from build123d import *

# Parameters (mm, degrees)
F0_R          = 6.35
F1_DEPTH      = 25.4
F2_W          = 19.05
F2_H          = 9.525
F3_DEPTH      = 25.401
F3_DEPTH_BACK = 25.401


with BuildPart() as f1:
    # F0 (on Top) → F1 (new body)
    with BuildSketch(Plane.XY):
        with BuildLine():
            Line((-34.925, -25.4), (34.925, -25.4))
            ThreePointArc((34.925, -25.4), (37.170064, -24.470064), (38.1, -22.225))
            Line((38.1, -22.225), (38.1, 22.225))
            ThreePointArc((38.1, 22.225), (37.170064, 24.470064), (34.925, 25.4))
            Line((34.925, 25.4), (-34.925, 25.4))
            ThreePointArc((-34.925, 25.4), (-37.170064, 24.470064), (-38.1, 22.225))
            Line((-38.1, 22.225), (-38.1, -22.225))
            ThreePointArc((-38.1, -22.225), (-37.170064, -24.470064), (-34.925, -25.4))
        make_face()
        Circle(F0_R, mode=Mode.SUBTRACT)
    extrude(amount=F1_DEPTH)

    # F2 (on Front) → F3 (cut, two sides)
    with BuildSketch(Plane.XZ) as f3_sk:
        with Locations((28.575, 20.6375)):
            Rectangle(F2_W, F2_H)
    extrude(amount=F3_DEPTH, mode=Mode.SUBTRACT)
    extrude(f3_sk.sketch, amount=-F3_DEPTH_BACK, mode=Mode.SUBTRACT)


solid = f1.part
Here's how the part is built. I have some questions about the finished solid (model axes, mm). A direction names the side the tool comes from. Give positions to 0.01 mm unless a question says otherwise; leave off trailing zeros. Order: outer loops, then holes, each group sorted by start corner. A loop starts at its lowest first (then second) coordinate and runs counter-clockwise, first axis right, second up. Notation, with made-up numbers: (71, 35) -> (85, 35) arc R19 cw to (85, 58) -> close; hole circle Ø4 at (-9, 80.5). An arc over 180 degrees is marked (long way). One line per item, written item: value. Start each with the question number.
1. Imagine slicing it at D-D, the plane y = -11. List the corners of the cut face in (x, z) for me (3 decimals).
2. Imagine slicing it at B-B, the plane y = 0. List the corners of the cut face in (x, z) for me (3 decimals).
3. For faces 5 (the face through (37.15, -24.49, 7.83)), 6 (the face through (19.05, 0, 21)), which set-ups out of +Z, -Z, +X, -X, +Y, -Y let a thin tool reach every point of the face, with its end or its side?
4. Will these pins go through, and if not, where does the flat tip stop? pin 1 Ø3 at (y, z) = (2.5, 20.5) entering from +X; pin 2 Ø9.5 at (x, y) = (25.5, -1.5) entering from +Z (3 decimals); pin 3 Ø4 at (x, z) = (21.5, 18.5) entering from -Y.
5. Imagine slicing it at C-C, the plane x = 5. List the corners of the cut face in (y, z) for me, plus the area to 3 significant figures.
6. We'd pull the mould along X, two halves only. Please class faces 1 (the face through (38.1, 0, 8)), 2 (the face through (-1.38, -6.2, 12.52)), 3 (the face through (-37.15, 24.49, 12.52)), 4 (the face through (-10, 0, 25.4)): released by +X, released by -X, zero draft, split by the parting line, or undercut.
7. I need wall thicknesses on probe 1 along Y at (x, z) = (0, 19.75); probe 2 along X at (y, z) = (22.5, 7.5); probe 3 along Z at (x, y) = (24.5, -3) (3 decimals). Which ranges of each line are inside material? Lowest first, please. Write a range as from..to.
8. Imagine slicing it at A-A, the plane z = 13. List the corners of the cut face in (x, y) for me (3 decimals).
Values follow:
1. outline: (-38.1, 0) -> (38.1, 0) -> (38.1, 15.875) -> (19.05, 15.875) -> (19.05, 25.4) -> (-38.1, 25.4) -> close
2. outline: (-38.1, 0) -> (-6.35, 0) -> (-6.35, 25.4) -> (-38.1, 25.4) -> close; (6.35, 0) -> (38.1, 0) -> (38.1, 15.875) -> (19.05, 15.875) -> (19.05, 25.4) -> (6.35, 25.4) -> close
3. face 5: +Z, -Z, +X, -Y
3. face 6: +Z, +X, +Y, -Y
4. pin 1: stops at x = 19.05
4. pin 2: stops at z = 15.875
4. pin 3: passes through
5. outline: (-25.4, 0) -> (-3.91, 0) -> (-3.91, 25.4) -> (-25.4, 25.4) -> close; (3.91, 0) -> (25.4, 0) -> (25.4, 25.4) -> (3.91, 25.4) -> close
5. area: 1,090 mm2
6. face 1: released by +X
6. face 2: undercut
6. face 3: released by -X
6. face 4: zero draft
7. probe 1: y = -25.4..-6.35, 6.35..25.4
7. probe 2: x = -38.09..38.09
7. probe 3: z = 0..15.875
8. outline: (-38.1, -22.225) arc R3.175 ccw to (-34.925, -25.4) -> (34.925, -25.4) arc R3.175 ccw to (38.1, -22.225) -> (38.1, 22.225) arc R3.175 ccw to (34.925, 25.4) -> (-34.925, 25.4) arc R3.175 ccw to (-38.1, 22.225) -> close; hole circle Ø12.7 at (0, 0)
